from build123d import *

# Parameters (mm, degrees)
F0_W     = 25.4
F0_H     = 3.175
F0_W_2   = 1.5875
F0_H_2   = 11.1125
F1_DEPTH = 6.35


with BuildPart() as f1:
    # F0 (on Top) → F1 (new body)
    with BuildSketch(Plane.XY):
        with Locations((-17.4625, -12.7)):
            Rectangle(F0_W, F0_H)
        with Locations((-3.96875, -5.55625)):
            Rectangle(F0_W_2, F0_H_2)
        Polygon((-3.175, -14.2875), (-3.175, -11.1125), (-4.7625, -11.1125), (-4.7625, -14.2875), (-4.7625, -25.4), (-3.175, -25.4), align=None)
        with Locations((-2.38125, -12.7)):
            Rectangle(F0_W_2, F0_H)
        Polygon((0, -25.4), (0, 0), (-1.5875, 0), (-1.5875, -11.1125), (-1.5875, -14.2875), (-1.5875, -25.4), align=None)
    extrude(amount=F1_DEPTH)


solid = f1.part
Can you work these out from the model? Positions are in its coordinate system, mm. A direction names the side the tool comes from. Coordinates: 2 decimals unless noted, no trailing zeros. Loops run counter-clockwise (first coordinate to the right, second up) from the corner with the lowest first, then second, coordinate; pieces in that order, holes last. Notation, with made-up numbers: (55.25, 7.5) - (60.25, 7.5) arc R14 cw to (60.25, 22.5) - close; hole circle Ø3 at (76.5, -14.5). An arc over 180 degrees is marked (long way). Put each result on its own line as item: value. Start each with the question number.
Item 1: Suppose I cut it at C-C (x = -22). Please give me the cut outline in (y, z).
Item 2: If we mould it in two halves opening along X, with no side actions, what happens to faces 1 (the face through (-4.762, -6, 3)), 2 (the face through (-4, 0, 3)), 3 (the face through (-1.588, -5, 3))? For each: +X half, -X half, draft (parallel to the pull), parting line (faces both ways), or undercut.
Item 3: If I drill on line 1 along X through (y, z) = (-18, 0.5) (1 decimal); line 2 along Y through (x, z) = (-14, 3.25), over which ranges is the centre line in solid material (lowest first)?
Item 4: Suppose I cut it at B-B (z = 3.25). Please give me the cut outline in (x, y) (1 decimal).
Item 5: Which directions (+Z, -Z, +X, -X, +Y, -Y) give clear straight access to the entire face, cutting with the end or side of a thin tool? Please do faces 4 (the face through (-1, -25.4, 3)), 5 (the face through (-18, -11.112, 3)), 6 (the face through (-4.762, -20, 3)), 7 (the face through (-2, -11.112, 3)), 8 (the face through (-2, -14.288, 3)).
Item 6: For pin 1 (3 mm diameter, centred on x = -23, z = 2.5, fed in from +Y), with a flat end and sliding along its axis, tell me the tip position at first contact or that it passes through.
Here are the results:
1. outline: (-14.29, 0) - (-11.11, 0) - (-11.11, 6.35) - (-14.29, 6.35) - close
2. face 1: -X half
2. face 2: draft
2. face 3: undercut
3. line 1: -4.8 to -3.2, -1.6 to 0
3. line 2: -14.29 to -11.11
4. outline: (-30.2, -14.3) - (-4.8, -14.3) - (-4.8, -25.4) - (-3.2, -25.4) - (-3.2, -14.3) - (-1.6, -14.3) - (-1.6, -25.4) - (0, -25.4) - (0, 0) - (-1.6, 0) - (-1.6, -11.1) - (-3.2, -11.1) - (-3.2, 0) - (-4.8, 0) - (-4.8, -11.1) - (-30.2, -11.1) - close
5. face 4: +Z, -Z, +X, -X, -Y
5. face 5: +Z, -Z, -X, +Y
5. face 6: +Z, -Z, -X, -Y
5. face 7: +Z, -Z, +Y
5. face 8: +Z, -Z, -Y
6. pin 1: y = -11.11
